The model under review builds one solid part; all positions refer to its coordinate system, in mm. Round coordinates to 2 decimals unless told otherwise and drop trailing zeros. Loops run counter-clockwise (first coordinate to the right, second up) from the corner with the lowest first, then second, coordinate; pieces in that order, holes last. Notation, with made-up numbers: (4.25, 75.25) -> (63.25, 75.25) arc R30 cw to (63.25, 106.25) -> close; hole circle Ø3 at (-24, 72.5). An arc over 180 degrees is marked (long way). Use a Markdown table: item, result. Add a question column.
1) Consider section B-B on x = -33. Give the boundary of the cut face in (y, z), plus the area to 3 significant figures.
2) Consider section A-A on z = 1.15. Give the boundary of the cut face in (x, y) (3 decimals).
3) Insertion check: pin 1 (3 mm diameter, centred on x = -18, y = 26, fed in from -Z); pin 2 (0.8 mm diameter, centred on y = 31.5, z = 0.5, fed in from -X) (3 decimals). Each pin has a flat end and moves straight along its axis. Give the tip position at first contact, or say it passes through.
4) Consider section C-C on y = 21. Give the boundary of the cut face in (x, z), plus the area to 3 significant figures.
5) Mouldability with a two-part tool opening along Y and no side actions: class faces 1 (the cylindrical face through (33.38, 21.73, 0.79)), 2 (the flat face through (-1, 1, 1.6)), 3 (the cylindrical face through (23.602, 28.239, 0.811)) as released by +Y, released by -Y, zero draft, split by the parting line, or undercut.
6) Wall thickness on probe 1 along Y at (x, z) = (-20.5, 0.9) (3 decimals); probe 2 along X at (y, z) = (30.5, 0.55) (3 decimals); probe 3 along X at (y, z) = (33, 1.25) (3 decimals): over which ranges is each line inside the solid? List them lowest first.
from build123d import *

# Parameters (mm, degrees)
F1_DEPTH = 1.6
F2_R     = 2
F3_DEPTH = 25


with BuildPart() as f1:
    # F0 (on Top) → F1 (new body)
    with BuildSketch(Plane.XY):
        with BuildLine():
            Line((30.875, 38.735), (-30.875, 38.735))
            Line((-30.875, 38.735), (-30.875, 27.685))
            ThreePointArc((-30.875, 27.685), (-33.314801, 21.794801), (-39.205, 19.355))
            Line((-39.205, 19.355), (-39.205, -19.355))
            ThreePointArc((-39.205, -19.355), (-33.314801, -21.794801), (-30.875, -27.685))
            Line((-30.875, -27.685), (-30.875, -38.735))
            Line((-30.875, -38.735), (30.875, -38.735))
            Line((30.875, -38.735), (30.875, -27.685))
            ThreePointArc((30.875, -27.685), (33.314801, -21.794801), (39.205, -19.355))
            Line((39.205, -19.355), (39.205, 19.355))
            ThreePointArc((39.205, 19.355), (33.314801, 21.794801), (30.875, 27.685))
            Line((30.875, 27.685), (30.875, 38.735))
        make_face()
    extrude(amount=F1_DEPTH)

    # F2 (on face) → F3 (cut)
    with BuildSketch(Plane.XY.offset(1.6)):
        with Locations((-21.755, 29.005)):
            Circle(F2_R)
        with Locations((21.755, 29.005)):
            Circle(F2_R)
        with Locations((-21.755, -29.005)):
            Circle(F2_R)
        with Locations((21.755, -29.005)):
            Circle(F2_R)
    extrude(amount=-F3_DEPTH, mode=Mode.SUBTRACT)


solid = f1.part
Result set:
| question | item | result |
|---|---|---|
| 1 | outline | (-22.13, 0) -> (22.13, 0) -> (22.13, 1.6) -> (-22.13, 1.6) -> close |
| 1 | area | 70.8 mm2 |
| 2 | outline | (-39.205, -19.355) arc R8.33 cw to (-30.875, -27.685) -> (-30.875, -38.735) -> (30.875, -38.735) -> (30.875, -27.685) arc R8.33 cw to (39.205, -19.355) -> (39.205, 19.355) arc R8.33 cw to (30.875, 27.685) -> (30.875, 38.735) -> (-30.875, 38.735) -> (-30.875, 27.685) arc R8.33 cw to (-39.205, 19.355) -> close; hole circle Ø4 at (-21.755, -29.005); hole circle Ø4 at (-21.755, 29.005); hole circle Ø4 at (21.755, -29.005); hole circle Ø4 at (21.755, 29.005) |
| 3 | pin 1 | z = 0 |
| 3 | pin 2 | x = -30.875 |
| 4 | outline | (-34.24, 0) -> (34.24, 0) -> (34.24, 1.6) -> (-34.24, 1.6) -> close |
| 4 | area | 110 mm2 |
| 5 | face 1 | released by +Y |
| 5 | face 2 | zero draft |
| 5 | face 3 | undercut |
| 6 | probe 1 | -38.735 to -30.562, -27.448 to 27.448, 30.562 to 38.735 |
| 6 | probe 2 | -30.875 to -23.084, -20.426 to 20.426, 23.084 to 30.875 |
| 6 | probe 3 | -30.875 to 30.875 |
